from build123d import *

# Parameters (mm, degrees)
CUT_EXTRUDE_1_DEPTH = 1.1


with BuildPart() as part:
    # Эскиз1 → Повернуть1 (revolve)
    with BuildSketch(Plane.XY, mode=Mode.PRIVATE) as revolve_1_sk:
        with BuildLine():
            Line((0, 0), (0, 2.05))
            Line((0, 2.05), (0.2, 2.25))
            Line((0.2, 2.25), (2.3, 2.25))
            Line((2.3, 2.25), (2.5, 2.05))
            Line((2.5, 2.05), (2.5, 1.45))
            ThreePointArc((2.5, 1.45), (2.558578644, 1.308578644), (2.7, 1.25))
            Line((2.7, 1.25), (12, 1.25))
            Line((12, 1.25), (12.5, 0.75))
            Line((12.5, 0.75), (12.5, 0))
            Line((12.5, 0), (0, 0))
        make_face()
    revolve(revolve_1_sk.sketch.rotate(Axis((0, 0, 0), (-1, 0, 0)), 90), axis=Axis((0, 0, 0), (-1, 0, 0)))

    # Эскиз2 → Вырез-Вытянуть1 (cut)
    with BuildSketch(Plane.ZY):
        Polygon((0, 1.154700538), (-1, 0.577350269), (-1, -0.577350269), (0, -1.154700538), (1, -0.577350269), (1, 0.577350269), align=None)
    extrude(amount=-CUT_EXTRUDE_1_DEPTH, mode=Mode.SUBTRACT)


solid = part.part
Part model, mm, in its own coordinate system. A direction names the side the tool comes from. Coordinates: 2 decimals unless noted, no trailing zeros. Loops run counter-clockwise (first coordinate to the right, second up) from the corner with the lowest first, then second, coordinate; pieces in that order, holes last. Notation, with made-up numbers: M -9.5,42.5 L 35.5,42.5 A26 cw 35.5,78.5 Z; hole C 69,9 d6. An arc over 180 degrees is marked long. Use a Markdown table: item, result. Add a question column.
Q1. Cut at B-B (x = 4). Write the cut outline in (y, z), and give its area (3 significant figures).
Q2. Mould opens along Z. For faces 4 (the cylindrical face through (7.42, -0.05, 1.25)), 5 (the flat face through (0, 1, 1)), 6 (the flat face through (0.5, 0, -1)) say: +Z half, -Z half, draft (parallel to the pull), parting line (faces both ways), or undercut.
Q3. Which spindle directions (+Z, -Z, +X, -X, +Y, -Y) get a long thin tool onto all of the face, cutting with end or side? Do faces 1 (the flat face through (2.5, 1.34, -0.88)), 2 (the flat face through (0.54, -0.87, 0.49)), 3 (the flat face through (12.5, 0, 0)). Say none if no direction does.
Q4. Pin check, flat tip, straight feed: P1, Ø2, axis at x = 7.5, y = -0.5, coming from the -Z side. Stop position of the tip, or through.
Q5. Probe L1, parallel to X at y = 0.4, z = 0.15; L2, parallel to X at y = 1.5, z = 0.8; L3, parallel to Y at x = 10.25, z = -0.05. List the from-to ranges inside material, lowest first.
Q6. Cut at A-A (y = 0). Write the cut outline in (x, z), and give its area (3 significant figures).
Worked out:
| question | item | result |
|---|---|---|
| 1 | outline | C 0,0 d2.5 |
| 1 | area | 4.91 mm2 |
| 2 | face 4 | parting line |
| 2 | face 5 | draft |
| 2 | face 6 | undercut |
| 3 | face 1 | +X |
| 3 | face 2 | -X |
| 3 | face 3 | +Z, -Z, +X, +Y, -Y |
| 4 | P1 | stops at z = -1.25 |
| 5 | L1 | x = 1.1 to 12.5 |
| 5 | L2 | x = 0 to 2.5 |
| 5 | L3 | y = -1.25 to 1.25 |
| 6 | outline | M 0,-2.05 L 0.2,-2.25 L 2.3,-2.25 L 2.5,-2.05 L 2.5,-1.45 A0.2 cw 2.7,-1.25 L 12,-1.25 L 12.5,-0.75 L 12.5,0.75 L 12,1.25 L 2.7,1.25 A0.2 cw 2.5,1.45 L 2.5,2.05 L 2.3,2.25 L 0.2,2.25 L 0,2.05 L 0,1 L 1.1,1 L 1.1,-1 L 0,-1 Z |
| 6 | area | 33.7 mm2 |
